CAD build for the part. Positions are in the model's coordinates, mm. A direction names the side the tool comes from. Round coordinates to 2 decimals unless told otherwise and drop trailing zeros. Loops run counter-clockwise (first coordinate to the right, second up) from the corner with the lowest first, then second, coordinate; pieces in that order, holes last. Notation, with made-up numbers: M 78.5,52.25 L 83.5,52.25 A36 cw 83.5,89.25 Z; hole C 40,-2.5 d11. An arc over 180 degrees is marked long. Use a Markdown table: item, result. Add a question column.
(1) Band-saw the part on B-B, the plane y = 147. Write the cut outline in (x, z) (1 decimal), and give its area (3 significant figures).
(2) Two-plate mould, pull along X, no slides. Class faces 1 (the face through (192, 95, 15.875)), 2 (the face through (-3.175, 97, 0)), 3 (the face through (0, 97, 2)), 4 (the face through (182.562, 95, 0)): released by +X, released by -X, zero draft, split by the parting line, or undercut.
(3) Wall check: L1, parallel to X at y = 140, z = -4 (1 decimal); L2, parallel to X at y = 28.5, z = 13.5; L3, parallel to Y at x = 150.5, z = 9.25. Give the ranges that are in metal, low to high.
(4) Band-saw the part on C-C, the plane x = 157. Write the cut outline in (y, z).
(5) Flat gauge pins, fed straight in: P1, Ø7.5, axis at y = 68, z = 0.5, coming from the -X side (3 decimals); P2, Ø1.6, axis at x = 110, y = 191.5, coming from the +Z side; P3, Ø4, axis at y = 20, z = 5, coming from the +X side. Where does each tip first touch, or does it go through?
(6) Which spindle directions (+Z, -Z, +X, -X, +Y, -Y) get a long thin tool onto all of the face, cutting with end or side? Do faces 5 (the face through (88, 188.912, 0)), 6 (the face through (-14, 95, 12.7)), 7 (the face through (194, 95, 12.7)), 8 (the face through (-2, 0, 8)). Say none if no direction does.
(7) Band-saw the part on A-A, the plane z = 9.25. Write the cut outline in (x, y) (1 decimal), and give its area (3 significant figures).
from build123d import *

# Parameters (mm, degrees)
BOSS_EXTRUDE1_DEPTH = 12.7
SKETCH2_W           = 3.175
SKETCH2_H           = 192.0875
BOSS_EXTRUDE2_DEPTH = 25.4


with BuildPart() as part:
    # Sketch1 → Boss-Extrude1 (new body, symmetric)
    with BuildSketch(Plane.XY):
        Polygon((0, 0), (0, 188.9125), (179.3875, 188.9125), (179.3875, 0), (182.5625, 0), (182.5625, 192.0875), (-3.175, 192.0875), (-3.175, 0), align=None)
    extrude(amount=BOSS_EXTRUDE1_DEPTH, both=True)

    # Sketch2 → Boss-Extrude2 (add)
    with BuildSketch(Plane(origin=(0, 0, 0), x_dir=(0, 0, -1), z_dir=(1, 0, 0))):
        with Locations((-14.2875, 96.04375)):
            Rectangle(SKETCH2_W, SKETCH2_H)
    boss_extrude2 = extrude(amount=-BOSS_EXTRUDE2_DEPTH)

    # Mirror1: Boss-Extrude2 across plane
    add(boss_extrude2.mirror(Plane(origin=(89.69375, 0, 0), x_dir=(0, 0, 1), z_dir=(1, 0, 0))))


solid = part.part
Return value:
| question | item | result |
|---|---|---|
| 1 | outline | M -25.4,12.7 L -3.2,12.7 L -3.2,-12.7 L 0,-12.7 L 0,15.9 L -25.4,15.9 Z; M 179.4,-12.7 L 182.6,-12.7 L 182.6,12.7 L 204.8,12.7 L 204.8,15.9 L 179.4,15.9 Z |
| 1 | area | 323 mm^2 |
| 2 | face 1 | zero draft |
| 2 | face 2 | released by -X |
| 2 | face 3 | undercut |
| 2 | face 4 | released by +X |
| 3 | L1 | -3.2 to 0, 179.4 to 182.6 |
| 3 | L2 | -25.4 to 0, 179.39 to 204.79 |
| 3 | L3 | 188.91 to 192.09 |
| 4 | outline | M 188.91,-12.7 L 192.09,-12.7 L 192.09,12.7 L 188.91,12.7 Z |
| 5 | P1 | x = -3.175 |
| 5 | P2 | z = 12.7 |
| 5 | P3 | x = 182.56 |
| 6 | face 5 | +Z, -Z, -Y |
| 6 | face 6 | -Z, -X, +Y, -Y |
| 6 | face 7 | -Z, +X, +Y, -Y |
| 6 | face 8 | +Z, -Z, +X, -X, -Y |
| 7 | outline | M -3.2,0 L 0,0 L 0,188.9 L 179.4,188.9 L 179.4,0 L 182.6,0 L 182.6,192.1 L -3.2,192.1 Z |
| 7 | area | 1,790 mm^2 |
